from build123d import *

# Parameters (mm, degrees)
CROQUIS1_R              = 2.5
SALIENTE_EXTRUIR1_DEPTH = 480
CUT_EXTRUDE1_DEPTH      = 47
CUT_EXTRUDE1_DEPTH_BACK = 46
SKETCH2_W               = 830
SKETCH2_H               = 37.339467532


with BuildPart() as part:
    # Croquis1 → Saliente-Extruir1 (new body)
    with BuildSketch(Plane.XY):
        with BuildLine():
            Line((-4.6, 10), (-3.1, 8.5))
            Line((-3.1, 8.5), (-3.1, 8.2))
            Line((-3.1, 8.2), (-5.5, 8.2))
            Line((-5.5, 8.2), (-5.5, 6.560660172))
            Line((-5.5, 6.560660172), (-2.84, 3.900660172))
            Line((-2.84, 3.900660172), (0, 3.900660172))
            Line((0, 3.900660172), (2.84, 3.900660172))
            Line((2.84, 3.900660172), (5.5, 6.560660172))
            Line((5.5, 6.560660172), (5.5, 8.2))
            Line((5.5, 8.2), (3.1, 8.2))
            Line((3.1, 8.2), (3.1, 8.5))
            Line((3.1, 8.5), (4.6, 10))
            Line((4.6, 10), (9.25, 10))
            ThreePointArc((9.25, 10), (9.780330086, 9.780330086), (10, 9.25))
            Line((10, 9.25), (10, 4.6))
            Line((10, 4.6), (8.5, 3.1))
            Line((8.5, 3.1), (8.2, 3.1))
            Line((8.2, 3.1), (8.2, 5.5))
            Line((8.2, 5.5), (6.560660172, 5.5))
            Line((6.560660172, 5.5), (3.900660172, 2.84))
            Line((3.900660172, 2.84), (3.900660172, 0))
            Line((3.900660172, 0), (3.900660172, -2.84))
            Line((3.900660172, -2.84), (6.560660172, -5.5))
            Line((6.560660172, -5.5), (8.2, -5.5))
            Line((8.2, -5.5), (8.2, -3.1))
            Line((8.2, -3.1), (8.5, -3.1))
            Line((8.5, -3.1), (10, -4.6))
            Line((10, -4.6), (10, -9.25))
            ThreePointArc((10, -9.25), (9.780330086, -9.780330086), (9.25, -10))
            Line((9.25, -10), (4.6, -10))
            Line((4.6, -10), (3.1, -8.5))
            Line((3.1, -8.5), (3.1, -8.2))
            Line((3.1, -8.2), (5.5, -8.2))
            Line((5.5, -8.2), (5.5, -6.560660172))
            Line((5.5, -6.560660172), (2.84, -3.900660172))
            Line((2.84, -3.900660172), (0, -3.900660172))
            Line((0, -3.900660172), (-2.84, -3.900660172))
            Line((-2.84, -3.900660172), (-5.5, -6.560660172))
            Line((-5.5, -6.560660172), (-5.5, -8.2))
            Line((-5.5, -8.2), (-3.1, -8.2))
            Line((-3.1, -8.2), (-3.1, -8.5))
            Line((-3.1, -8.5), (-4.6, -10))
            Line((-4.6, -10), (-9.25, -10))
            ThreePointArc((-9.25, -10), (-9.780330086, -9.780330086), (-10, -9.25))
            Line((-10, -9.25), (-10, -4.6))
            Line((-10, -4.6), (-8.5, -3.1))
            Line((-8.5, -3.1), (-8.2, -3.1))
            Line((-8.2, -3.1), (-8.2, -5.5))
            Line((-8.2, -5.5), (-6.560660172, -5.5))
            Line((-6.560660172, -5.5), (-3.900660172, -2.84))
            Line((-3.900660172, -2.84), (-3.900660172, 0))
            Line((-3.900660172, 0), (-3.900660172, 2.84))
            Line((-3.900660172, 2.84), (-6.560660172, 5.5))
            Line((-6.560660172, 5.5), (-8.2, 5.5))
            Line((-8.2, 5.5), (-8.2, 3.1))
            Line((-8.2, 3.1), (-8.5, 3.1))
            Line((-8.5, 3.1), (-10, 4.6))
            Line((-10, 4.6), (-10, 9.25))
            ThreePointArc((-10, 9.25), (-9.780330086, 9.780330086), (-9.25, 10))
            Line((-9.25, 10), (-4.6, 10))
        make_face()
        Circle(CROQUIS1_R, mode=Mode.SUBTRACT)
    extrude(amount=SALIENTE_EXTRUIR1_DEPTH)

    # Sketch2 → Cut-Extrude1 (cut, two sides: drawn at the far end of the back side and taken through both)
    with BuildSketch(Plane(origin=(0, 0, 0), x_dir=(0, 0, -1), z_dir=(1, 0, 0)).offset(-CUT_EXTRUDE1_DEPTH_BACK)):
        Rectangle(SKETCH2_W, SKETCH2_H)
    extrude(amount=CUT_EXTRUDE1_DEPTH + CUT_EXTRUDE1_DEPTH_BACK, mode=Mode.SUBTRACT)


solid = part.part
Read the model definition and answer for the solid it produces. Units are mm, in the model's axes. A direction names the side the tool comes from. Coordinates: 2 decimals unless noted, no trailing zeros. Loops run counter-clockwise (first coordinate to the right, second up) from the corner with the lowest first, then second, coordinate; pieces in that order, holes last. Notation, with made-up numbers: (32, 61.25) -> (67, 61.25) arc R16 ccw to (67, 91.25) -> close; hole circle Ø5 at (38.25, 15). An arc over 180 degrees is marked (long way). Write item = value, one per line. Start each with the question number.
1) Given P1, Ø2, axis at y = -0.5, z = 422, coming from the -X side; P2, Ø6, axis at x = 0.5, z = 456.5, coming from the -Y side; P3, Ø4.5, axis at y = -1, z = 434, coming from the +X side, each flat-ended and moving along its own axis, determine where each tip first touches the part or whether it passes through.
2) The mould has two halves that part along X. Classify faces 1 (the face through (5.5, -7, 447)), 2 (the face through (-7, -10, 447)), 3 (the face through (10, 7, 447)): pulls with the +X half, pulls with the -X half, needs draft (parallel to the pull), parting line crosses it, or undercut.
3) The part is cut by section A-A, the plane y = 0. Determine the outline of the cut face in (x, z), plus the area to 3 significant figures.
4) Find the intervals of material crossed by L1, parallel to X at y = -8.25, z = 470; L2, parallel to X at y = 0, z = 466, in increasing order. Write a range as from..to.
5) For faces 4 (the face through (3.901, 0, 447)), 5 (the face through (-9.3, -3.9, 447)), 6 (the face through (8.2, -4, 447)), 7 (the face through (-3.9, 9.3, 447)), 8 (the face through (0, -3.901, 447)), determine the directions among +Z, -Z, +X, -X, +Y, -Y from which every point of the face is accessible in a straight line to the end or side of a thin tool.
Result:
q1.P1 = -3.9
q1.P2 = -8.9
q1.P3 = 8.65
q2.face_1 = undercut
q2.face_2 = needs draft
q2.face_3 = pulls with the +X half
q3.outline = (-3.9, 415) -> (-2.5, 415) -> (-2.5, 480) -> (-3.9, 480) -> close; (2.5, 415) -> (3.9, 415) -> (3.9, 480) -> (2.5, 480) -> close
q3.area = 182 mm²
q4.L1 = -10..-3.1, 3.1..10
q4.L2 = -3.9..-2.5, 2.5..3.9
q5.face_4 = +Z, -Z, +X
q5.face_5 = +Z, -Z, -X
q5.face_6 = +Z, -Z
q5.face_7 = +Z, -Z, +Y
q5.face_8 = +Z, -Z, -Y
